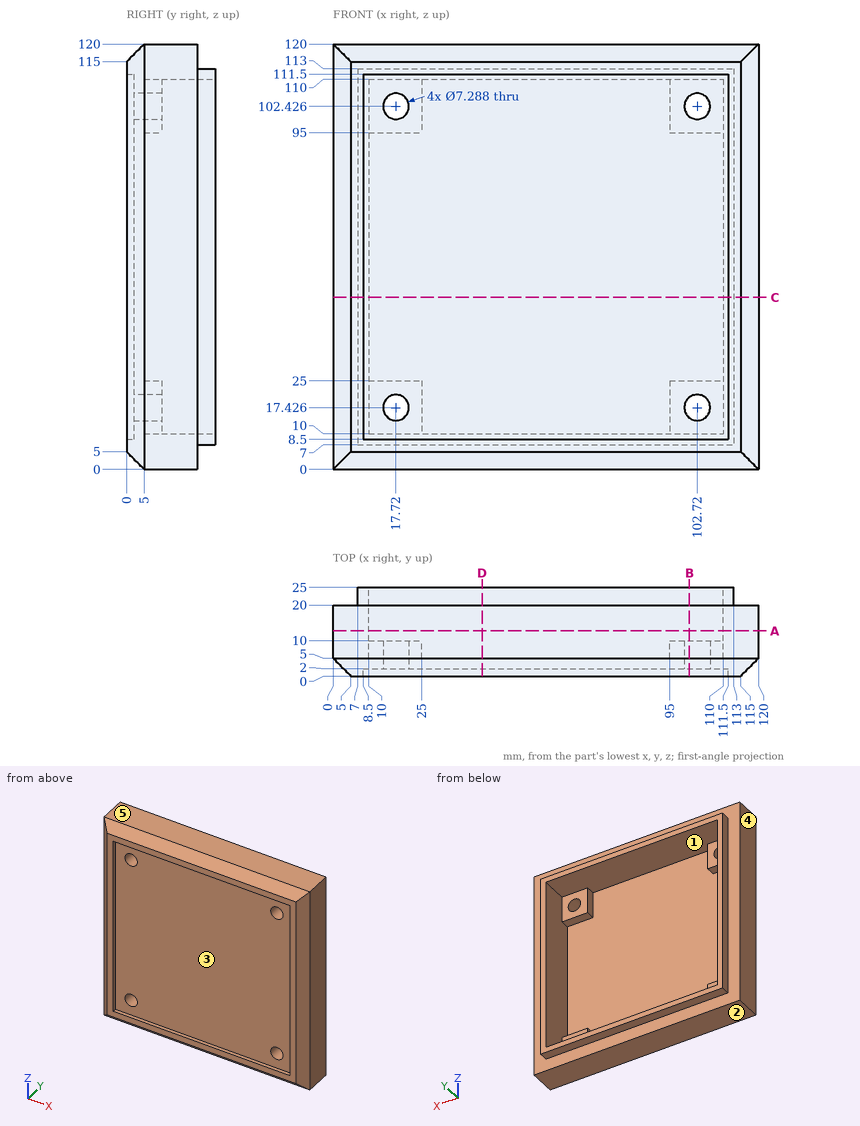
For this review, use the dimensioned drawing (mm, ordinates from the lowest corner) and the shaded views. A direction names the side the tool comes from. Give positions to 0.01 mm unless a question says otherwise; leave off trailing zeros. Loops run counter-clockwise (first coordinate to the right, second up) from the corner with the lowest first, then second, coordinate; pieces in that order, holes last.
Item 1: Draft analysis for pull direction Z (two halves, no side actions). For the marked faces 3, 4 and 5, state which applies: +Z half, -Z half, draft (parallel to the pull), parting line (faces both ways), or undercut.
Item 2: Take a section at D-D, the plane x = 42. State the section outline as (y, z) points, and give its area (3 significant figures).
Item 3: Take a section at A-A, the plane y = 12.75. State the section outline as (x, z) points.
Item 4: Take a section at B-B, the plane x = 100.5. Give the number of separate pieces and of enclosed holes in the cut face.
Item 5: Insertion check: pin 1 (4.5 mm diameter, centred on x = 102.72, z = 102.43, fed in from +Y); pin 2 (5 mm diameter, centred on y = 22, z = 32.5, fed in from +X); pin 3 (12 mm diameter, centred on x = 100.5, z = 18, fed in from +Y); pin 4 (2.5 mm diameter, centred on y = 22, z = 53, fed in from -X). Each pin has a flat end and moves straight along its axis. Give the tip position at first contact, or say it passes through.
Item 6: For line 1 along X through (y, z) = (11.75, 68.5); line 2 along X through (y, z) = (24.25, 90), list the stretches that pass through material, from the lowest coordinate up.
Item 7: Tool access review of the marked faces 1 and 2: name each direction out of +Z, -Z, +X, -X, +Y, -Y from which nothing blocks a thin tool from reaching the whole face with its end or side.
Item 8: Take a section at C-C, the plane z = 48.5. State the section outline as (x, y) points.
Calculated:
1. face 3: undercut
1. face 4: draft
1. face 5: +Z half
2. outline: (0, 5) - (5, 0) - (20, 0) - (20, 7) - (25, 7) - (25, 10) - (5, 10) - (5, 110) - (25, 110) - (25, 113) - (20, 113) - (20, 120) - (5, 120) - (0, 115) - (0, 111.5) - (2, 111.5) - (2, 8.5) - (0, 8.5) - close
2. area: 699 mm2
3. outline: (0, 0) - (120, 0) - (120, 120) - (0, 120) - close; hole (10, 10) - (110, 10) - (110, 110) - (10, 110) - close
4. separate pieces: 3
4. enclosed holes: 0
5. pin 1: passes through
5. pin 2: stops at x = 120
5. pin 3: stops at y = 10
5. pin 4: stops at x = 7
6. line 1: x = 0 to 10, 110 to 120
6. line 2: x = 7 to 10, 110 to 113
7. face 1: +Y
7. face 2: -Z, +X, -X, +Y, -Y
8. outline: (0, 5) - (5, 0) - (8.5, 0) - (8.5, 2) - (111.5, 2) - (111.5, 0) - (115, 0) - (120, 5) - (120, 20) - (113, 20) - (113, 25) - (110, 25) - (110, 5) - (10, 5) - (10, 25) - (7, 25) - (7, 20) - (0, 20) - close
